from build123d import *

# Parameters (mm, degrees)
F0_W     = 25.4
F0_H     = 88.9
F1_DEPTH = 25.4
F2_W     = 25.4
F2_H     = 25.4
F3_DEPTH = 38.1
F4_W     = 25.4
F4_H     = 63.5
F5_DEPTH = 12.7
F6_R     = 19.05
F7_DEPTH = 25.4


with BuildPart() as f1:
    # F0 (on Top) → F1 (new body)
    with BuildSketch(Plane.XY):
        with Locations((-99.183585, -28.025017)):
            Rectangle(F0_W, F0_H)
        with BuildLine():
            Line((-42.033585, 16.424983), (-86.483585, 16.424983))
            Line((-86.483585, 16.424983), (-86.483585, -72.475017))
            Line((-86.483585, -72.475017), (-42.033585, -72.475017))
            ThreePointArc((-42.033585, -72.475017), (2.416415, -28.025017), (-42.033585, 16.424983))
        make_face()
    extrude(amount=F1_DEPTH)

    # F2 (on face) → F3 (join)
    with BuildSketch(Plane.XY.offset(25.4)):
        with Locations((-99.183585, 3.724983)):
            Rectangle(F2_W, F2_H)
    extrude(amount=F3_DEPTH)

    # F4 (on face) → F5 (join)
    with BuildSketch(Plane.XY.offset(25.4)):
        with Locations((-99.183585, -40.725017)):
            Rectangle(F4_W, F4_H)
    extrude(amount=F5_DEPTH)

    # F6 (on face) → F7 (cut)
    with BuildSketch(Plane.XY.offset(25.4)):
        with Locations((-42.033585, -28.025017)):
            Circle(F6_R)
    extrude(amount=-F7_DEPTH, mode=Mode.SUBTRACT)


solid = f1.part
Part model, mm, in its own coordinate system. A direction names the side the tool comes from. Give positions to 0.01 mm unless a question says otherwise; leave off trailing zeros. Write each loop counter-clockwise with the first axis right and the second up, starting at its lowest first coordinate (ties: lowest second). Pieces come first, ordered by that corner, then holes.
1) Cut at D-D on z = 54.5. Write the cut outline in (x, y), then the cut area to 3 significant figures.
Resolved:
outline: (-111.88, -8.98) - (-86.48, -8.98) - (-86.48, 16.42) - (-111.88, 16.42) - close
area: 645 mm2
2) Pin check, flat tips, straight feed: pin 1 (5 mm diameter, centred on x = -40, y = -1, fed in from -Z); pin 2 (7.5 mm diameter, centred on x = -98, z = 55.5, fed in from -Y) (3 decimals); pin 3 (19 mm diameter, centred on y = -31.5, z = 44.5, fed in from +X); pin 4 (3 mm diameter, centred on x = -69.5, y = -58.5, fed in from +Z). Stop position of each tip, or through.
Resolved:
pin 1: stops at z = 0
pin 2: stops at y = -8.975
pin 3: stops at x = -86.48
pin 4: stops at z = 25.4
3) Probe L1, parallel to X at y = -30, z = 5.5; L2, parallel to Z at x = -3, y = -10.5; L3, parallel to Y at x = -102.5, z = 43.5. List the from-to ranges inside material, lowest first.
Resolved:
L1: x = -111.88 to -60.98, -23.09 to 2.37
L2: z = 0 to 25.4
L3: y = -8.98 to 16.42
4) Cut at A-A on y = -35. Write the cut outline in (x, z).
Resolved:
outline: (-111.88, 0) - (-59.76, 0) - (-59.76, 25.4) - (-86.48, 25.4) - (-86.48, 38.1) - (-111.88, 38.1) - close; (-24.31, 0) - (1.87, 0) - (1.87, 25.4) - (-24.31, 25.4) - close
5) Two-plate mould, pull along Y, no slides. Class faces 4 (the face through (-86.484, -19, 36)), 5 (the face through (-46.163, -46.622, 12.878)), 6 (the face through (2.406, -29.002, 12.522)): released by +Y, released by -Y, zero draft, split by the parting line, or undercut.
Resolved:
face 4: zero draft
face 5: undercut
face 6: split by the parting line
6) Cut at C-C on z = 12.5. Write the cut outline in (x, y).
Resolved:
outline: (-111.88, -72.48) - (-42.03, -72.48) arc R44.45 ccw to (-42.03, 16.42) - (-111.88, 16.42) - close; hole circle Ø38.1 at (-42.03, -28.03)
7) Cut at B-B on x = -31. Write the cut outline in (y, z), then the cut area to 3 significant figures.
Resolved:
outline: (-71.08, 0) - (-43.55, 0) - (-43.55, 25.4) - (-71.08, 25.4) - close; (-12.5, 0) - (15.03, 0) - (15.03, 25.4) - (-12.5, 25.4) - close
area: 1,400 mm2
8) Which spindle directions (+Z, -Z, +X, -X, +Y, -Y) get a long thin tool onto all of the face, cutting with end or side? Do faces 1 (the face through (-62, -27, 25.4)), 2 (the face through (-99, -8.975, 51)), 3 (the face through (-68, -27, 0)). Say none if no direction does.
Resolved:
face 1: +Z, +X, +Y, -Y
face 2: +Z, +X, -X, -Y
face 3: -Z, +X, -X, +Y, -Y
